```python
from build123d import *

# Parameters (mm, degrees)
SKETCH1_W           = 59
SKETCH1_H           = 8
SKETCH1_R           = 1.5
BOSS_EXTRUDE1_DEPTH = 6
SKETCH2_W           = 47
SKETCH2_H           = 7
CUT_EXTRUDE1_DEPTH  = 15


with BuildPart() as part:
    # Sketch1 → Boss-Extrude1 (new body)
    with BuildSketch(Plane.XY):
        Rectangle(SKETCH1_W, SKETCH1_H)
        with Locations((-26.5, 0)):
            Circle(SKETCH1_R, mode=Mode.SUBTRACT)
        with Locations((-15, 0)):
            Circle(SKETCH1_R, mode=Mode.SUBTRACT)
        with Locations((15, 0)):
            Circle(SKETCH1_R, mode=Mode.SUBTRACT)
        with Locations((26.5, 0)):
            Circle(SKETCH1_R, mode=Mode.SUBTRACT)
    extrude(amount=BOSS_EXTRUDE1_DEPTH)

    # Sketch2 → Cut-Extrude1 (cut)
    with BuildSketch(Plane(origin=(0, 4, 0), x_dir=(-1, 0, 0), z_dir=(0, 1, 0))):
        Rectangle(SKETCH2_W, SKETCH2_H)
    extrude(amount=-CUT_EXTRUDE1_DEPTH, mode=Mode.SUBTRACT)


solid = part.part
```
Work out the finished part from the listing and answer in its coordinate system (mm). A direction names the side the tool comes from. Give positions to 0.01 mm unless a question says otherwise; leave off trailing zeros. Loops run counter-clockwise (first coordinate to the right, second up) from the corner with the lowest first, then second, coordinate; pieces in that order, holes last. Notation, with made-up numbers: (80.5, 45) -> (99.5, 45) arc R11 ccw to (99.5, 51) -> close; hole circle Ø7 at (32, 51). An arc over 180 degrees is marked (long way). One line per question, with ' | ' between items. Start each with the question number.
1) Section D-D, the plane z = 5 is taken. Determine the outline of the cut face in (x, y), then the cut area to 3 significant figures.
2) Section B-B, the plane x = 26.5 is taken. Determine the outline of the cut face in (y, z).
3) Each of these flat-tipped pins is pushed along its axis until it touches: pin 1 (4 mm diameter, centred on x = -15, y = 0, fed in from -Z); pin 2 (1.8 mm diameter, centred on x = 15, y = 0, fed in from -Z). Where does it stop, or does it pass through?
4) For faces 1 (the face through (29.5, 0, 3)), 2 (the face through (0, 0, 3.5)), determine the directions among +Z, -Z, +X, -X, +Y, -Y from which every point of the face is accessible in a straight line to the end or side of a thin tool.
5) Section C-C, the plane y = 0 is taken. Determine the outline of the cut face in (x, z), then the cut area to 4 significant figures.
6) Straight lines are drawn through the part: L1, parallel to X at y = 2.25, z = 1.8; L2, parallel to Y at x = -26.5, z = 2.1; L3, parallel to X at y = -1, z = 1.2. For each, find the intervals that lie inside material, in ascending order.
7) Section A-A, the plane z = 2.35 is taken. Determine the outline of the cut face in (x, y).
Resolved:
1) outline: (-29.5, -4) -> (29.5, -4) -> (29.5, 4) -> (-29.5, 4) -> close; hole circle Ø3 at (-26.5, 0); hole circle Ø3 at (-15, 0); hole circle Ø3 at (15, 0); hole circle Ø3 at (26.5, 0) | area: 444 mm2
2) outline: (-4, 0) -> (-1.5, 0) -> (-1.5, 6) -> (-4, 6) -> close; (1.5, 0) -> (4, 0) -> (4, 6) -> (1.5, 6) -> close
3) pin 1: z = 3.5 | pin 2: through
4) face 1: +Z, -Z, +X, +Y, -Y | face 2: -Z, +Y, -Y
5) outline: (-29.5, 0) -> (-28, 0) -> (-28, 6) -> (-29.5, 6) -> close; (-25, 0) -> (-23.5, 0) -> (-23.5, 3.5) -> (-16.5, 3.5) -> (-16.5, 6) -> (-25, 6) -> close; (-13.5, 3.5) -> (13.5, 3.5) -> (13.5, 6) -> (-13.5, 6) -> close; (16.5, 3.5) -> (23.5, 3.5) -> (23.5, 0) -> (25, 0) -> (25, 6) -> (16.5, 6) -> close; (28, 0) -> (29.5, 0) -> (29.5, 6) -> (28, 6) -> close | area: 138.5 mm2
6) L1: -29.5 to -23.5, 23.5 to 29.5 | L2: -4 to -1.5, 1.5 to 4 | L3: -29.5 to -27.62, -25.38 to -23.5, 23.5 to 25.38, 27.62 to 29.5
7) outline: (-29.5, -4) -> (-23.5, -4) -> (-23.5, 4) -> (-29.5, 4) -> close; (23.5, -4) -> (29.5, -4) -> (29.5, 4) -> (23.5, 4) -> close; hole circle Ø3 at (-26.5, 0); hole circle Ø3 at (26.5, 0)
